Check sheet for the drawn part. Datum: minimum x, y, z corner. Units: mm. A direction names the side the tool comes from. Coordinates: 2 decimals unless noted, no trailing zeros. Write each loop counter-clockwise with the first axis right and the second up, starting at its lowest first coordinate (ties: lowest second). Pieces come first, ordered by that corner, then holes. Notation, with made-up numbers: M 28,-33 L 35,-33 A33 cw 35,4 Z; hole C 45.25,-2.5 d5. An arc over 180 degrees is marked long. Answer as CSV lines item,"result". Start each with the question number.
Q1. Sectioned sample at A-A, the plane y = 12.75. Record the cut outline in (x, z), then the cut area to 3 significant figures.
Q2. Mould release check, pull along Z, two halves, no side actions. Record for the marked faces 1, 2, 3 and 4: pulls with the +Z half, pulls with the -Z half, needs draft (parallel to the pull), parting line crosses it, or undercut.
Q3. Sectioned sample at C-C, the plane z = 47.5. Record the cut outline in (x, y), then the cut area to 3 significant figures.
Q4. Access from +Z, -Z, +X, -X, +Y, -Y to the whole of each face (thin tool, end or side, straight path). Record for the marked faces 5 and 6.
Q5. Sectioned sample at D-D, the plane x = 73. Record the cut outline in (y, z), then the cut area to 3 significant figures.
Q6. Sectioned sample at B-B, the plane y = 7.5. Record the cut outline in (x, z).
Q7. Depth check by flat-ended pin: pin 1 Ø12 at (x, z) = (12.5, 47.5) entering from -Y; pin 2 Ø1.5 at (y, z) = (8, 58) entering from -X (1 decimal); pin 3 Ø1.5 at (y, z) = (7, 58.5) entering from +X (1 decimal); pin 4 Ø4.5 at (x, z) = (11.5, 14) entering from +Y. Enter the tip coordinate at first touch or a pass-through.
Q8. Thickness scan on line 1 along Z through (x, y) = (67.5, 11.5); line 2 along Z through (x, y) = (12.5, 12); line 3 along Z through (x, y) = (67.5, 8.75). Record the ranges inside material, lowest first. Write a range as from..to.
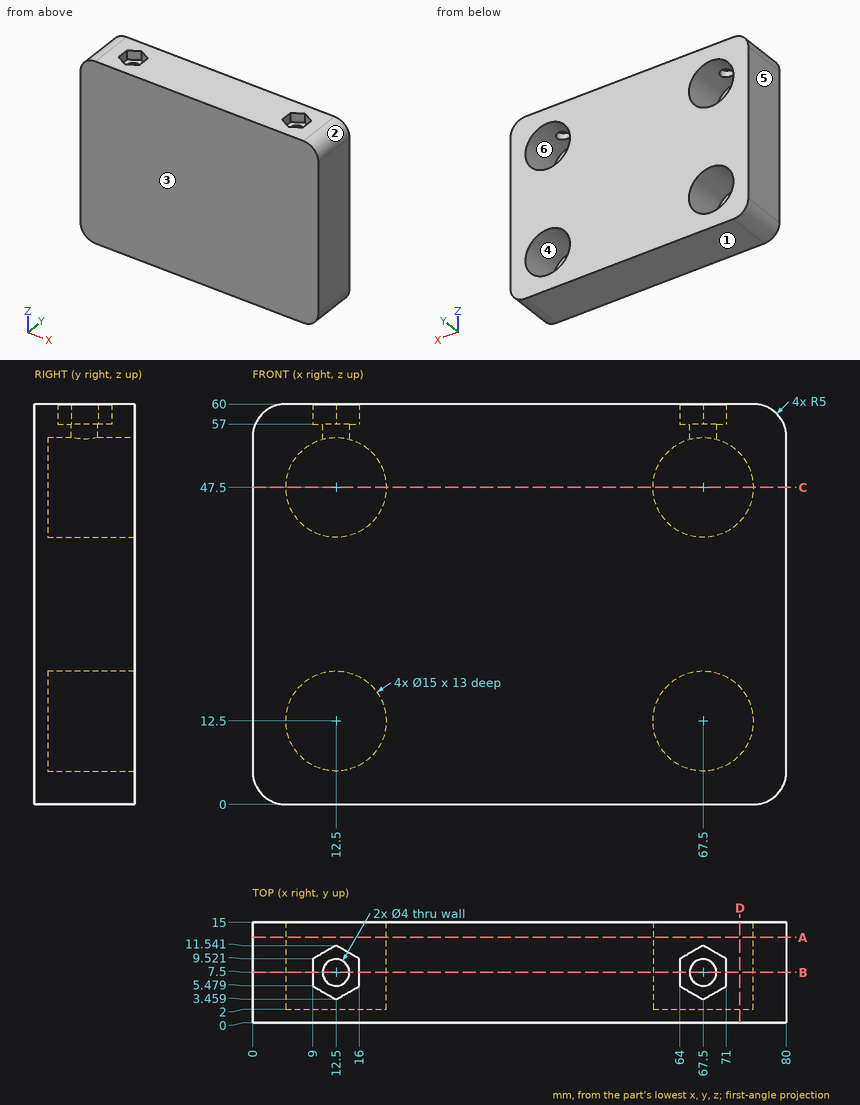
Output:
1,outline,"M 0,5 A5 ccw 5,0 L 75,0 A5 ccw 80,5 L 80,55 A5 ccw 75,60 L 5,60 A5 ccw 0,55 Z; hole C 12.5,12.5 d15; hole C 12.5,47.5 d15; hole C 67.5,12.5 d15; hole C 67.5,47.5 d15"
1,area,"4,070 mm^2"
2,face 1,"pulls with the -Z half"
2,face 2,"pulls with the +Z half"
2,face 3,"needs draft"
2,face 4,"undercut"
3,outline,"M 0,0 L 80,0 L 80,15 L 75,15 L 75,2 L 60,2 L 60,15 L 20,15 L 20,2 L 5,2 L 5,15 L 0,15 Z"
3,area,"810 mm^2"
4,face 5,"+Z, -Z, -X, +Y, -Y"
4,face 6,"+Y"
5,outline,"M 0,0 L 15,0 L 15,7.4 L 2,7.4 L 2,17.6 L 15,17.6 L 15,42.4 L 2,42.4 L 2,52.6 L 15,52.6 L 15,60 L 0,60 Z"
5,area,"635 mm^2"
6,outline,"M 0,5 A5 ccw 5,0 L 75,0 A5 ccw 80,5 L 80,55 A5 ccw 75,60 L 71,60 L 71,57 L 69.5,57 L 69.5,54.73 A7.5 cw long 65.5,54.73 L 65.5,57 L 64,57 L 64,60 L 16,60 L 16,57 L 14.5,57 L 14.5,54.73 A7.5 cw long 10.5,54.73 L 10.5,57 L 9,57 L 9,60 L 5,60 A5 ccw 0,55 Z; hole C 12.5,12.5 d15; hole C 67.5,12.5 d15"
7,pin 1,"stops at y = 0"
7,pin 2,"stops at x = 0.5"
7,pin 3,"stops at x = 79.2"
7,pin 4,"stops at y = 2"
8,line 1,"z = 0..5, 20..40, 55..57"
8,line 2,"z = 0..5, 20..40, 55..60"
8,line 3,"z = 0..5, 20..40"
